The listing builds one solid part. Answer for the finished solid, in the listing's coordinates (mm). Coordinates: 2 decimals unless noted, no trailing zeros. Write each loop counter-clockwise with the first axis right and the second up, starting at its lowest first coordinate (ties: lowest second). Pieces come first, ordered by that corner, then holes.
from build123d import *

# Parameters (mm, degrees)
EXTRUDE_1_DEPTH     = 4
FILLET_1_R          = 2
SKETCH_2_R          = 2.5
CUT_EXTRUDE_1_DEPTH = 83.474238402
SKETCH_3_R          = 11
CUT_EXTRUDE_2_DEPTH = 83.474238402


with BuildPart() as part:
    # 草图1 → 凸台-拉伸1 (new body)
    with BuildSketch(Plane.XY):
        Polygon((45, 0), (-45, 0), (-45, 14), (-17, 14), (-17, 55), (-45, 55), (-45, 69), (45, 69), (45, 55), (17, 55), (17, 14), (45, 14), align=None)
    extrude(amount=EXTRUDE_1_DEPTH)

    # 圆角1
    fillet_1_edges = [part.edges().sort_by_distance(p)[0] for p in [
        (-17, 14, 2),
        (-17, 55, 2),
        (17, 55, 2),
        (17, 14, 2),
    ]]
    fillet(fillet_1_edges, radius=FILLET_1_R)

    # 草图2 → 切除-拉伸1 (cut, through all)
    with BuildSketch(Plane.XY.offset(4)):
        with Locations((-37.5, 61.5)):
            Circle(SKETCH_2_R)
        with Locations(Location((37.5, 61.5, 0), (0, 0, 180))):
            Circle(SKETCH_2_R)
        with Locations((-12.5, 61.5)):
            Circle(SKETCH_2_R)
        with Locations(Location((12.5, 61.5, 0), (0, 0, 180))):
            Circle(SKETCH_2_R)
        with Locations((-37.5, 7.5)):
            Circle(SKETCH_2_R)
        with Locations(Location((37.5, 7.5, 0), (0, 0, 180))):
            Circle(SKETCH_2_R)
        with Locations((-12.5, 7.5)):
            Circle(SKETCH_2_R)
        with Locations(Location((12.5, 7.5, 0), (0, 0, 180))):
            Circle(SKETCH_2_R)
    extrude(amount=-CUT_EXTRUDE_1_DEPTH, mode=Mode.SUBTRACT)

    # 草图3 → 切除-拉伸2 (cut, through all)
    with BuildSketch(Plane.XY.offset(4)):
        with Locations((0, 34.5)):
            Circle(SKETCH_3_R)
    extrude(amount=-CUT_EXTRUDE_2_DEPTH, mode=Mode.SUBTRACT)


solid = part.part
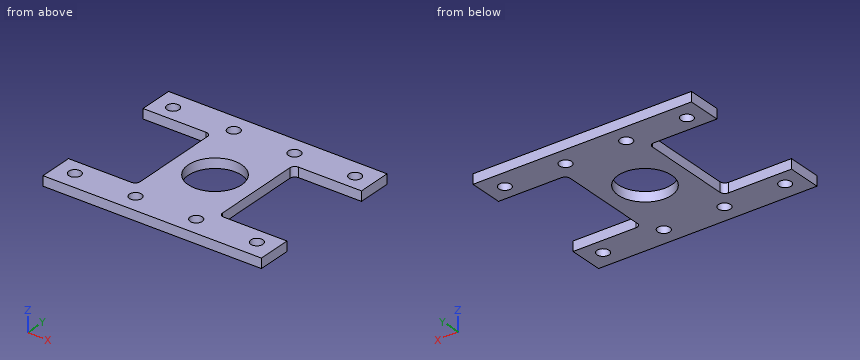
1. Section B-B on x = -37.5 is taken. Give the vertices of the cut face in (y, z), then the cut area to 3 significant figures.
Results found:
outline: (0, 0) - (5, 0) - (5, 4) - (0, 4) - close; (10, 0) - (14, 0) - (14, 4) - (10, 4) - close; (55, 0) - (59, 0) - (59, 4) - (55, 4) - close; (64, 0) - (69, 0) - (69, 4) - (64, 4) - close
area: 72.0 mm2
2. Section A-A on y = 61.5 is taken. Give the vertices of the cut face in (x, z).
Results found:
outline: (-45, 0) - (-40, 0) - (-40, 4) - (-45, 4) - close; (-35, 0) - (-15, 0) - (-15, 4) - (-35, 4) - close; (-10, 0) - (10, 0) - (10, 4) - (-10, 4) - close; (15, 0) - (35, 0) - (35, 4) - (15, 4) - close; (40, 0) - (45, 0) - (45, 4) - (40, 4) - close
3. Section C-C on z = 1.3 is taken. State how many separate pieces and enclosed holes the cut face has, then the cut area to 3 significant figures.
Results found:
separate pieces: 1
enclosed holes: 9
area: 3,380 mm2
4. Find the intervals of material crossed by L1, parallel to Y at x = -12.5, z = 1.05; L2, parallel to Y at x = 37.5, z = 2.7; L3, parallel to Y at x = -24, z = 1.75, in increasing order.
Results found:
L1: y = 0 to 5, 10 to 59, 64 to 69
L2: y = 0 to 5, 10 to 14, 55 to 59, 64 to 69
L3: y = 0 to 14, 55 to 69
5. Section D-D on y = 34.5 is taken. Give the vertices of the cut face in (x, z), then the cut area to 3 significant figures.
Results found:
outline: (-17, 0) - (-11, 0) - (-11, 4) - (-17, 4) - close; (11, 0) - (17, 0) - (17, 4) - (11, 4) - close
area: 48.0 mm2
